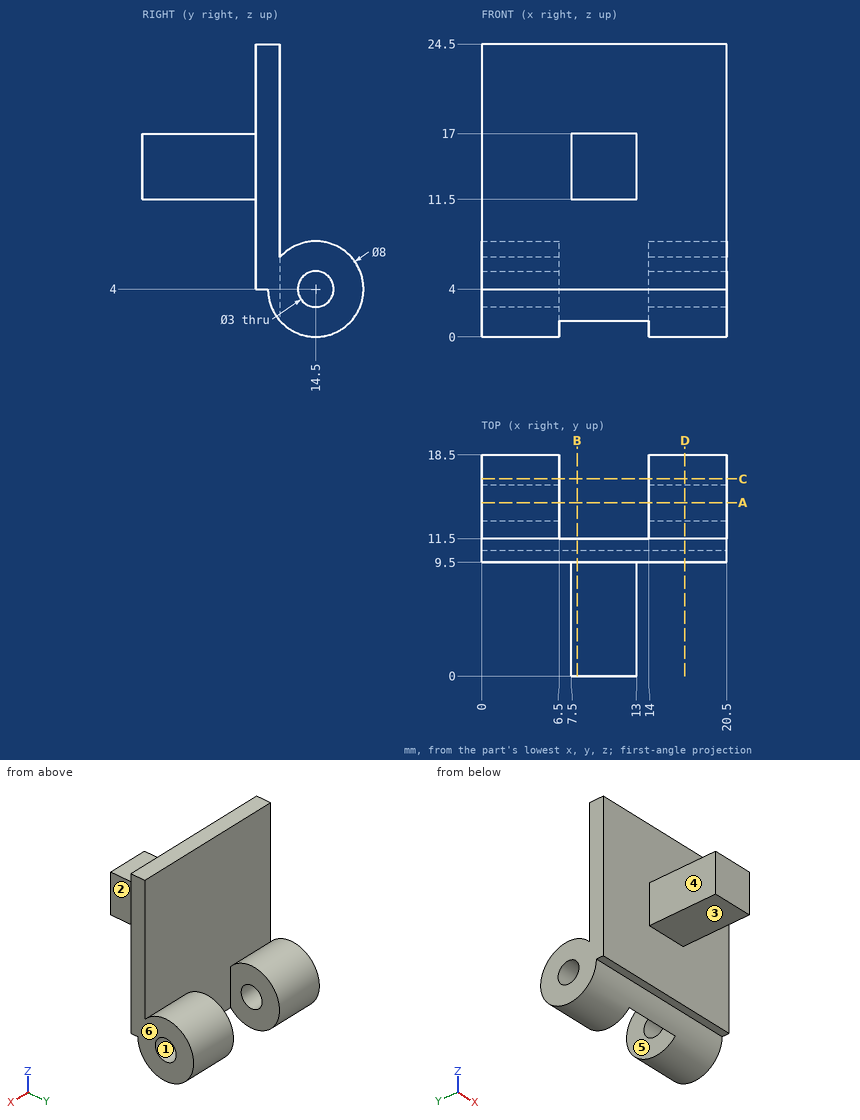
Answer from the drawing. Dimensions are ordinates in mm from the lowest x, y and z of the part. A direction names the side the tool comes from. Round coordinates to 2 decimals unless told otherwise and drop trailing zeros. Write each loop counter-clockwise with the first axis right and the second up, starting at its lowest first coordinate (ties: lowest second). Pieces come first, ordered by that corner, then holes. Notation, with made-up numbers: M 18,-36.75 L 49,-36.75 A19 ccw 49,-6.75 Z; hole C -4.75,61 d3. An arc over 180 degrees is marked long. Write each question's results on one line, items separated by ' | '. Start each with the question number.
Item 1: For a pull along Z with two mould halves and no side action, classify the marked faces 1, 2 and 3 as pulls with the +Z half, pulls with the -Z half, needs draft (parallel to the pull), parting line crosses it, or undercut.
Item 2: A cutting plane is placed at D-D on x = 17. Write down the section's boundary in (y, z).
Item 3: For the marked faces 4, 5 and 6, determine the directions among +Z, -Z, +X, -X, +Y, -Y from which every point of the face is accessible in a straight line to the end or side of a thin tool.
Item 4: A cutting plane is placed at C-C on y = 16.5. Write down the section's boundary in (x, z), and give its area (3 significant figures).
Item 5: A cutting plane is placed at B-B on x = 8. Write down the section's boundary in (y, z).
Item 6: Flat-ended cylindrical pins translate along their axes: pin 1 Ø2.5 at (y, z) = (14.5, 4) entering from -X; pin 2 Ø3 at (x, y) = (10.5, 3.5) entering from -Z; pin 3 Ø3 at (x, z) = (3, 18.5) entering from +Y; pin 4 Ø4.5 at (x, y) = (10, 5) entering from +Z. Find the tip coordinate at first contact, or state that the pin passes through.
Item 7: Straight lines are drawn through the part: L1, parallel to X at y = 12.25, z = 2.25; L2, parallel to Z at x = 1.5, y = 14.5; L3, parallel to Y at x = 2.75, z = 21.25. For each, find the intervals that lie inside material, in ascending order. Write a range as [from, to].
Item 8: A cutting plane is placed at A-A on y = 14.5. Write down the section's boundary in (x, z).
Check sheet entries:
1) face 1: undercut | face 2: needs draft | face 3: pulls with the -Z half
2) outline: M 9.5,4 L 10.5,4 A4 ccw long 11.5,6.65 L 11.5,24.5 L 9.5,24.5 Z; hole C 14.5,4 d3
3) face 4: +Z, -Z, -X, -Y | face 5: +Z, -Z, +Y | face 6: +Z, -Z, +X, +Y, -Y
4) outline: M 0,0.54 L 6.5,0.54 L 6.5,7.46 L 0,7.46 Z; M 14,0.54 L 20.5,0.54 L 20.5,7.46 L 14,7.46 Z | area: 90.1 mm²
5) outline: M 0,11.5 L 9.5,11.5 L 9.5,4 L 10.5,4 A4 ccw 11.5,1.35 L 11.5,24.5 L 9.5,24.5 L 9.5,17 L 0,17 Z
6) pin 1: through | pin 2: z = 11.5 | pin 3: y = 11.5 | pin 4: z = 17
7) L1: [0, 6.5], [14, 20.5] | L2: [0, 2.5], [5.5, 8] | L3: [9.5, 11.5]
8) outline: M 0,0 L 6.5,0 L 6.5,2.5 L 0,2.5 Z; M 0,5.5 L 6.5,5.5 L 6.5,8 L 0,8 Z; M 14,0 L 20.5,0 L 20.5,2.5 L 14,2.5 Z; M 14,5.5 L 20.5,5.5 L 20.5,8 L 14,8 Z
